```python
from build123d import *

# Parameters (mm, degrees)
SKETCH1_W           = 221
SKETCH1_H           = 45
BOSS_EXTRUDE1_DEPTH = 5
SKETCH2_W           = 211
SKETCH2_H           = 25
CUT_EXTRUDE1_DEPTH  = 2.5
SKETCH3_R           = 8
CUT_EXTRUDE2_DEPTH  = 2.5
SKETCH6_W           = 221
SKETCH6_H           = 45
SKETCH6_W_2         = 216
SKETCH6_H_2         = 40
BOSS_EXTRUDE3_DEPTH = 30
SKETCH7_W           = 7
SKETCH7_H           = 7.5
BOSS_EXTRUDE4_DEPTH = 17.5
SKETCH9_R           = 1
CUT_EXTRUDE3_DEPTH  = 6
SKETCH10_W          = 30
SKETCH10_H          = 35
BOSS_EXTRUDE5_DEPTH = 7
SKETCH11_R          = 1
CUT_EXTRUDE4_DEPTH  = 6


with BuildPart() as part:
    # Sketch1 → Boss-Extrude1 (new body)
    with BuildSketch(Plane(origin=(0, 0, 0), x_dir=(1, 0, 0), z_dir=(0, 1, 0))):
        Rectangle(SKETCH1_W, SKETCH1_H)
    extrude(amount=BOSS_EXTRUDE1_DEPTH)

    # Sketch2 → Cut-Extrude1 (cut)
    with BuildSketch(Plane(origin=(0, 5, 0), x_dir=(1, 0, 0), z_dir=(0, 1, 0))):
        Rectangle(SKETCH2_W, SKETCH2_H)
    extrude(amount=-CUT_EXTRUDE1_DEPTH, mode=Mode.SUBTRACT)

    # Sketch3 → Cut-Extrude2 (cut)
    with BuildSketch(Plane(origin=(0, 2.5, 0), x_dir=(1, 0, 0), z_dir=(0, 1, 0))):
        with Locations(Location((-53, 0, 0), (0, 0, 270))):
            Circle(SKETCH3_R)
        with Locations(Location((53, 0, 0), (0, 0, 270))):
            Circle(SKETCH3_R)
    extrude(amount=-CUT_EXTRUDE2_DEPTH, mode=Mode.SUBTRACT)

    # Sketch6 → Boss-Extrude3 (add)
    with BuildSketch(Plane(origin=(0, 5, 0), x_dir=(1, 0, 0), z_dir=(0, 1, 0))):
        Rectangle(SKETCH6_W, SKETCH6_H)
        Rectangle(SKETCH6_W_2, SKETCH6_H_2, mode=Mode.SUBTRACT)
    extrude(amount=BOSS_EXTRUDE3_DEPTH)

    # Sketch7 → Boss-Extrude4 (add)
    with BuildSketch(Plane(origin=(0, 5, 0), x_dir=(1, 0, 0), z_dir=(0, 1, 0))):
        with Locations((-89, 16.25)):
            Rectangle(SKETCH7_W, SKETCH7_H)
        with Locations((-89, -16.25)):
            Rectangle(SKETCH7_W, SKETCH7_H)
        with Locations((-16.5, 16.25)):
            Rectangle(SKETCH7_W, SKETCH7_H)
        with Locations((-16.5, -16.25)):
            Rectangle(SKETCH7_W, SKETCH7_H)
        with Locations((16.5, 16.25)):
            Rectangle(SKETCH7_W, SKETCH7_H)
        with Locations((16.5, -16.25)):
            Rectangle(SKETCH7_W, SKETCH7_H)
        with Locations((89, 16.25)):
            Rectangle(SKETCH7_W, SKETCH7_H)
        with Locations((89, -16.25)):
            Rectangle(SKETCH7_W, SKETCH7_H)
    extrude(amount=BOSS_EXTRUDE4_DEPTH)

    # Sketch9 → Cut-Extrude3 (cut)
    with BuildSketch(Plane(origin=(0, 22.5, 0), x_dir=(1, 0, 0), z_dir=(0, 1, 0))):
        with Locations(Location((-89, 16, 0), (0, 0, 270))):
            Circle(SKETCH9_R)
        with Locations(Location((-89, -16, 0), (0, 0, 270))):
            Circle(SKETCH9_R)
        with Locations(Location((-16.5, 16, 0), (0, 0, 270))):
            Circle(SKETCH9_R)
        with Locations(Location((-16.5, -16, 0), (0, 0, 270))):
            Circle(SKETCH9_R)
        with Locations(Location((16.5, 16, 0), (0, 0, 270))):
            Circle(SKETCH9_R)
        with Locations(Location((16.5, -16, 0), (0, 0, 270))):
            Circle(SKETCH9_R)
        with Locations(Location((89, 16, 0), (0, 0, 270))):
            Circle(SKETCH9_R)
        with Locations(Location((89, -16, 0), (0, 0, 270))):
            Circle(SKETCH9_R)
    extrude(amount=-CUT_EXTRUDE3_DEPTH, mode=Mode.SUBTRACT)

    # Sketch10 → Boss-Extrude5 (add)
    with BuildSketch(Plane.XY.offset(22.5)):
        with Locations((0, 17.5)):
            Rectangle(SKETCH10_W, SKETCH10_H)
    extrude(amount=BOSS_EXTRUDE5_DEPTH)

    # Sketch11 → Cut-Extrude4 (cut)
    with BuildSketch(Plane.XY.offset(29.5)):
        with Locations((-8, 28)):
            Circle(SKETCH11_R)
        with Locations((8, 28)):
            Circle(SKETCH11_R)
        with Locations((-8, 7)):
            Circle(SKETCH11_R)
        with Locations((8, 7)):
            Circle(SKETCH11_R)
    extrude(amount=-CUT_EXTRUDE4_DEPTH, mode=Mode.SUBTRACT)


solid = part.part
```
Could you check a few things on this model? Use its own coordinates, in mm. A direction names the side the tool comes from. Round coordinates to 2 decimals unless told otherwise and drop trailing zeros. Loops run counter-clockwise (first coordinate to the right, second up) from the corner with the lowest first, then second, coordinate; pieces in that order, holes last. Notation, with made-up numbers: (-15.5, -38) -> (40.5, -38) arc R25 cw to (40.5, -21) -> close; hole circle Ø2 at (39, -13). An arc over 180 degrees is marked (long way). Put each result on its own line as item: value.
Q1. Please list where these lines run through material, in increasing order: line 1 (Y direction, x = 8, z = 28.1); line 2 (Z direction, x = -89, y = 20); line 3 (X direction, y = 21.5, z = -14). Write a range as from..to.
Checks:
line 1: 0..6, 8..27, 29..35
line 2: -22.5..-17, -15..-12.5, 12.5..15, 17..22.5
line 3: -110.5..-108, -92.5..-85.5, -20..-13, 13..20, 85.5..92.5, 108..110.5
Q2. Thinking about a two-plate mould opening in X: for faces 5 (the flat face through (110.5, 17, 0)), 6 (the flat face through (-1, 35, 21)), 7 (the flat face through (13, 14, 16)), which applies, pulls with the +X half, pulls with the -X half, needs draft (parallel to the pull), parting line crosses it, or undercut?
Checks:
face 5: pulls with the +X half
face 6: needs draft
face 7: undercut
Q3. I want a section at B-B on x = -53. Write out the boundary of the cut face in (y, z).
Checks:
outline: (0, -22.5) -> (35, -22.5) -> (35, -20) -> (5, -20) -> (5, -12.5) -> (2.5, -12.5) -> (2.5, -8) -> (0, -8) -> close; (0, 8) -> (2.5, 8) -> (2.5, 12.5) -> (5, 12.5) -> (5, 20) -> (35, 20) -> (35, 22.5) -> (0, 22.5) -> close
Q4. Which directions (+Z, -Z, +X, -X, +Y, -Y) give clear straight access to the entire face, cutting with the end or side of a thin tool? Please do faces 1 (the flat face through (0, 18, 29.5)), 2 (the flat face through (15, 17, 26)), 3 (the flat face through (-108, 20, 0)), 4 (the flat face through (-63, 17, 22.5)).
Checks:
face 1: +Z, +X, -X, +Y, -Y
face 2: +Z, +X, +Y, -Y
face 3: +Y
face 4: +Z, -X, +Y, -Y
Q5. I want a section at D-D on x = -79.5. Write out the boundary of the cut face in (y, z).
Checks:
outline: (0, -22.5) -> (35, -22.5) -> (35, -20) -> (5, -20) -> (5, -12.5) -> (2.5, -12.5) -> (2.5, 12.5) -> (5, 12.5) -> (5, 20) -> (35, 20) -> (35, 22.5) -> (0, 22.5) -> close
Q6. For pin 1 Ø10.5 at (x, y) = (41.5, 21.5) entering from +Z; pin 2 Ø2 at (y, z) = (10.5, 24.5) entering from -X; pin 3 Ø1 at (x, y) = (8, 28) entering from +Z, each with a flat end and sliding along its axis, tell me the tip position at first contact or that it passes through.
Checks:
pin 1: z = 22.5
pin 2: x = -15
pin 3: z = 23.5
Q7. I want a section at C-C on y = 31. Write out the boundary of the cut face in (x, z).
Checks:
outline: (-110.5, -22.5) -> (110.5, -22.5) -> (110.5, 22.5) -> (15, 22.5) -> (15, 29.5) -> (-15, 29.5) -> (-15, 22.5) -> (-110.5, 22.5) -> close; hole (-108, -20) -> (108, -20) -> (108, 20) -> (-108, 20) -> close
Q8. I want a section at A-A on z = 0. Write out the boundary of the cut face in (x, y).
Checks:
outline: (-110.5, 0) -> (-61, 0) -> (-61, 2.5) -> (-105.5, 2.5) -> (-105.5, 5) -> (-108, 5) -> (-108, 35) -> (-110.5, 35) -> close; (-45, 0) -> (45, 0) -> (45, 2.5) -> (-45, 2.5) -> close; (61, 0) -> (110.5, 0) -> (110.5, 35) -> (108, 35) -> (108, 5) -> (105.5, 5) -> (105.5, 2.5) -> (61, 2.5) -> close
